For this review, take the finished solid that the model builds, in its own axes (mm). A direction names the side the tool comes from. Coordinates: 2 decimals unless noted, no trailing zeros. Write each loop counter-clockwise with the first axis right and the second up, starting at its lowest first coordinate (ties: lowest second). Pieces come first, ordered by that corner, then holes.
```python
from build123d import *

# Parameters (mm, degrees)
SKETCH_R     = 13.5
PAD_DEPTH    = 30
SKETCH001_R  = 12
PAD001_DEPTH = 30
SKETCH002_R  = 2.1
PAD002_DEPTH = 6.75
FILLET_R     = 0.5
FILLET001_R  = 0.5


with BuildPart() as part:
    # Sketch → Pad (new body)
    with BuildSketch(Plane.XY):
        Circle(SKETCH_R)
    extrude(amount=PAD_DEPTH)

    # Sketch001 (on Face2 of Pad) → Pad001 (join)
    with BuildSketch(Plane(origin=(0, 0, 0), x_dir=(1, 0, 0), z_dir=(0, 0, -1))):
        Circle(SKETCH001_R)
    extrude(amount=PAD001_DEPTH)

    # Sketch002 (on Face3 of Pad001) → Pad002 (join)
    with BuildSketch(Plane.XY.offset(30)):
        Circle(SKETCH002_R)
        with Locations((0, -8.9)):
            Circle(SKETCH002_R)
    extrude(amount=PAD002_DEPTH)

    # Fillet
    fillet_edges = [part.edges().sort_by_distance(p)[0] for p in [
        (-2.1, 0, 36.75),
    ]]
    fillet(fillet_edges, radius=FILLET_R)

    # Fillet001
    fillet001_edges = [part.edges().sort_by_distance(p)[0] for p in [
        (-2.1, -8.9, 36.75),
    ]]
    fillet(fillet001_edges, radius=FILLET001_R)


solid = part.part
```
Q1. Add section B-B (y = 0). State the section outline as (x, z) points, then the cut area to 3 significant figures.
Ans:
outline: (-13.5, 0) - (-12, 0) - (-12, -30) - (12, -30) - (12, 0) - (13.5, 0) - (13.5, 30) - (2.1, 30) - (2.1, 36.25) arc R0.5 ccw to (1.6, 36.75) - (-1.6, 36.75) arc R0.5 ccw to (-2.1, 36.25) - (-2.1, 30) - (-13.5, 30) - close
area: 1,560 mm2
Q2. Add section D-D (x = 11.25). State the section outline as (y, z) points, then the cut area to 3 significant figures.
Ans:
outline: (-7.46, 0) - (-4.18, 0) - (-4.18, -30) - (4.18, -30) - (4.18, 0) - (7.46, 0) - (7.46, 30) - (-7.46, 30) - close
area: 698 mm2
Q3. For probe 1 along Z at (x, y) = (-8, 3.5); probe 2 along X at (y, z) = (0, -15.5); probe 3 along Y at (x, z) = (-0.5, -7.5), list the stretches that pass through material, from the lowest coordinate up.
Ans:
probe 1: z = -30 to 30
probe 2: x = -12 to 12
probe 3: y = -11.99 to 11.99
Q4. Clearance check with flat-ended pins moving along their axes: pin 1 Ø3 at (y, z) = (7, 8.5) entering from +X; pin 2 Ø5 at (y, z) = (-2, -19.5) entering from +X; pin 3 Ø8 at (x, y) = (-9.5, 9) entering from +Z. State where each tip first meets the part, or that it passes through.
Ans:
pin 1: stops at x = 12.33
pin 2: stops at x = 12
pin 3: stops at z = 30
Q5. Draft analysis for pull direction Y (two halves, no side actions). For faces 1 (the cylindrical face through (-11.99, -0.53, -14.79)), 2 (the cylindrical face through (-0.273, -6.818, 33.081)), 3 (the flat face through (0, 0, -30)), state which applies: +Y half, -Y half, draft (parallel to the pull), parting line (faces both ways), or undercut.
Ans:
face 1: parting line
face 2: undercut
face 3: draft
Q6. Add section A-A (x = 0). State the section outline as (y, z) points.
Ans:
outline: (-13.5, 0) - (-12, 0) - (-12, -30) - (12, -30) - (12, 0) - (13.5, 0) - (13.5, 30) - (2.1, 30) - (2.1, 36.25) arc R0.5 ccw to (1.6, 36.75) - (-1.6, 36.75) arc R0.5 ccw to (-2.1, 36.25) - (-2.1, 30) - (-6.8, 30) - (-6.8, 36.25) arc R0.5 ccw to (-7.3, 36.75) - (-10.5, 36.75) arc R0.5 ccw to (-11, 36.25) - (-11, 30) - (-13.5, 30) - close
Q7. Add section C-C (z = -22). State the section outline as (x, y) points, then the cut area to 3 significant figures.
Ans:
outline: circle Ø24 at (0, 0)
area: 452 mm2
Q8. Tool access review of faces 4 (the cylindrical face through (2.003, 0.631, 33.081)), 5 (the flat face through (0, -9, 36.75)), 6 (the flat face through (-12, -2, 0)): name each direction out of +Z, -Z, +X, -X, +Y, -Y from which nothing blocks a thin tool from reaching the whole face with its end or side.
Ans:
face 4: +Z
face 5: +Z, +X, -X, +Y, -Y
face 6: -Z
